Read the model definition and answer for the solid it produces. Units are mm, in the model's axes. A direction names the side the tool comes from. Coordinates: 2 decimals unless noted, no trailing zeros. Write each loop counter-clockwise with the first axis right and the second up, starting at its lowest first coordinate (ties: lowest second). Pieces come first, ordered by that corner, then holes. Notation, with made-up numbers: (-12.5, 28.25) - (1.5, 28.25) arc R9 cw to (1.5, 45.25) - close; hole circle Ø9 at (43.5, 10.5). An arc over 180 degrees is marked (long way). Return JSON: item names as keys, results as strings.
```python
from build123d import *

# Parameters (mm, degrees)
BOSS_EXTRUDE1_DEPTH        = 2
M3_CLEARANCE_HOLE1_D       = 3.242
HOLE1_D                    = 10.1
SKETCHED_START             = 62.517190459
SKETCHED_BEND1_OUTLINE_W   = 2
SKETCHED_BEND1_OUTLINE_H   = 20.000000002
SKETCHED_BEND1_DEPTH       = 31.482809541
SKETCHED_START_2           = 60.939670459
SKETCHED_BEND1_2_OUTLINE_R = 5.05
SKETCHED_BEND1_2_DEPTH     = 0.021621314
SKETCHED_START_3           = 58.939670459
SKETCHED_BEND1_3_OUTLINE_R = 5.05
SKETCHED_BEND1_3_DEPTH     = 4
SKETCHED_START_4           = -10.000000001
SKETCHED_BEND1_4_DEPTH     = 20.000000002
CUT_EXTRUDE1_REACH         = 45.464


with BuildPart() as part:
    # Sketch5 → Boss-Extrude1 (new body)
    with BuildSketch(Plane(origin=(1.681750162, 0, 0), x_dir=(0, -1, 0), z_dir=(-1, 0, 0))):
        with BuildLine():
            Line((-35.93967046, 10.000000001), (-86.258661155, 10.000000001))
            Line((-86.258661155, 10.000000001), (-90.955360298, 5.303300858))
            ThreePointArc((-90.955360298, 5.303300858), (-93.152059438, 0), (-90.955360298, -5.303300858))
            Line((-90.955360298, -5.303300858), (-86.258661155, -10.000000001))
            Line((-86.258661155, -10.000000001), (-35.93967046, -10.000000001))
            ThreePointArc((-35.93967046, -10.000000001), (-33.818350116, -9.121320344), (-32.93967046, -7.000000001))
            Line((-32.93967046, -7.000000001), (-32.93967046, 7.000000001))
            ThreePointArc((-32.93967046, 7.000000001), (-33.818350116, 9.121320344), (-35.93967046, 10.000000001))
        make_face()
    extrude(amount=-BOSS_EXTRUDE1_DEPTH)

    # M3 Clearance Hole1 (through all)
    with Locations(Plane(origin=(3.681750162, 0, 0), x_dir=(0, 0, -1), z_dir=(1, 0, 0))):
        with Locations((0, 40.439670459), (0, 55.439670459)):
            Hole(M3_CLEARANCE_HOLE1_D / 2)

    # Hole1 (through all)
    with Locations(Plane.ZY.offset(-1.681750162)):
        with Locations((0, 85.65205944)):
            Hole(HOLE1_D / 2)

    # Sketched Bend1: read off the stored shape, not the designer's step
    # Sketched Bend1 outline → Sketched Bend1 (cut)
    with BuildSketch(Plane(origin=(0, 0, 0), x_dir=(1, 0, 0), z_dir=(0, 1, 0)).offset(SKETCHED_START)):
        with Locations((2.681750162, 0)):
            Rectangle(SKETCHED_BEND1_OUTLINE_W, SKETCHED_BEND1_OUTLINE_H)
    extrude(amount=SKETCHED_BEND1_DEPTH, mode=Mode.SUBTRACT)

    # Sketched Bend1 2 outline → Sketched Bend1 2 (add)
    with BuildSketch(Plane(origin=(0, 0, 0), x_dir=(1, 0, 0), z_dir=(0, 1, 0)).offset(SKETCHED_START_2)):
        with BuildLine():
            Line((1.681750162, 10.000000001), (-22.924851553, 10.000000001))
            Line((-22.924851553, 10.000000001), (-27.621550696, 5.303300858))
            ThreePointArc((-27.621550696, 5.303300858), (-29.818249837, 0), (-27.621550696, -5.303300858))
            Line((-27.621550696, -5.303300858), (-22.924851553, -10.000000001))
            Line((-22.924851553, -10.000000001), (1.681750162, -10.000000001))
            Line((1.681750162, -10.000000001), (1.681750162, 10.000000001))
        make_face()
        with Locations((-22.318249838, 0)):
            Circle(SKETCHED_BEND1_2_OUTLINE_R, mode=Mode.SUBTRACT)
    extrude(amount=SKETCHED_BEND1_2_DEPTH)

    # Sketched Bend1 3 outline → Sketched Bend1 3 (add)
    with BuildSketch(Plane(origin=(0, 0, 0), x_dir=(1, 0, 0), z_dir=(0, 1, 0)).offset(SKETCHED_START_3)):
        with BuildLine():
            Line((1.681750162, 10.000000001), (-22.924851553, 10.000000001))
            Line((-22.924851553, 10.000000001), (-27.621550696, 5.303300858))
            ThreePointArc((-27.621550696, 5.303300858), (-29.818249837, 0), (-27.621550696, -5.303300858))
            Line((-27.621550696, -5.303300858), (-22.924851553, -10.000000001))
            Line((-22.924851553, -10.000000001), (1.681750162, -10.000000001))
            Line((1.681750162, -10.000000001), (1.681750162, 10.000000001))
        make_face()
        with Locations((-22.318249838, 0)):
            Circle(SKETCHED_BEND1_3_OUTLINE_R, mode=Mode.SUBTRACT)
    extrude(amount=SKETCHED_BEND1_3_DEPTH)

    # Sketched Bend1 4 outline → Sketched Bend1 4 (cut)
    with BuildSketch(Plane.XY.offset(SKETCHED_START_4)):
        with BuildLine():
            Line((-0.318249838, 60.939670459), (-31, 60.939670459))
            Line((-31, 60.939670459), (-31, 58.939670459))
            Line((-31, 58.939670459), (1.681750162, 58.939670459))
            ThreePointArc((1.681750162, 58.939670459), (1.095963724, 60.353884021), (-0.318249838, 60.939670459))
        make_face()
        with BuildLine():
            Line((-31, 64), (-31, 62.939670452))
            Line((-31, 62.939670452), (-0.318249838, 62.939670459))
            ThreePointArc((-0.318249838, 62.939670459), (2.510177287, 61.768097584), (3.681750162, 58.939670459))
            Line((3.681750162, 58.939670459), (3.681750162, 62.517190459))
            Line((3.681750162, 62.517190459), (1.681750162, 62.517190459))
            Line((1.681750162, 62.517190459), (1.681750162, 64))
            Line((1.681750162, 64), (-31, 64))
        make_face()
    extrude(amount=SKETCHED_BEND1_4_DEPTH, mode=Mode.SUBTRACT)

    # Sketch15 → Cut-Extrude1 (cut, up to next)
    with BuildSketch(Plane(origin=(0, 62.939670459, 0), x_dir=(1, 0, 0), z_dir=(0, 1, 0)), mode=Mode.PRIVATE) as cut_extrude1_sk1:
        with BuildLine():
            Line((-21.068249838, 9.000000001), (-21.068249838, 10.000000001))
            Line((-21.068249838, 10.000000001), (-22.924851553, 10.000000001))
            Line((-22.924851553, 10.000000001), (-23.568249838, 9.356601716))
            Line((-23.568249838, 9.356601716), (-23.568249838, 9.000000001))
            Line((-23.568249838, 9.000000001), (-22.943249838, 8.375000001))
            ThreePointArc((-22.943249838, 8.375000001), (-22.318249838, 8.116116524), (-21.693249838, 8.375000001))
            Line((-21.693249838, 8.375000001), (-21.068249838, 9.000000001))
        make_face()
    cut_extrude1_tool1 = extrude(cut_extrude1_sk1.sketch, amount=-CUT_EXTRUDE1_REACH, mode=Mode.PRIVATE) & part.part
    # Sketch15 → Cut-Extrude1 (cut, up to next)
    with BuildSketch(Plane(origin=(0, 62.939670459, 0), x_dir=(1, 0, 0), z_dir=(0, 1, 0)), mode=Mode.PRIVATE) as cut_extrude1_sk2:
        with BuildLine():
            Line((-21.068249838, -9.000000001), (-21.693249838, -8.375000001))
            ThreePointArc((-21.693249838, -8.375000001), (-22.318249838, -8.116116524), (-22.943249838, -8.375000001))
            Line((-22.943249838, -8.375000001), (-23.568249838, -9.000000001))
            Line((-23.568249838, -9.000000001), (-23.568249838, -9.356601716))
            Line((-23.568249838, -9.356601716), (-22.924851553, -10.000000001))
            Line((-22.924851553, -10.000000001), (-21.068249838, -10.000000001))
            Line((-21.068249838, -10.000000001), (-21.068249838, -9.000000001))
        make_face()
    cut_extrude1_tool2 = extrude(cut_extrude1_sk2.sketch, amount=-CUT_EXTRUDE1_REACH, mode=Mode.PRIVATE) & part.part
    add(cut_extrude1_tool1.solids().sort_by_distance((-22.260131, 62.93967, -9.16246))[0], mode=Mode.SUBTRACT)
    add(cut_extrude1_tool2.solids().sort_by_distance((-22.260131, 62.93967, 9.16246))[0], mode=Mode.SUBTRACT)


solid = part.part
```
(1) Flat-ended cylindrical pins translate along their axes: P1, Ø1.1, axis at y = 62, z = 9.5, coming from the -X side; P2, Ø6, axis at y = 44, z = -1.5, coming from the -X side; P3, Ø2, axis at x = -5.5, z = 6.5, coming from the -Y side. Find the tip coordinate at first contact, or state that the pin passes through.
Answer:
{"P1": "x = -23.97", "P2": "x = 1.68", "P3": "y = 60.94"}
(2) A cutting plane is placed at C-C (z = 3.5). Determine the outline of the cut face in (x, y).
Answer:
{"outline": "(-28.95, 60.94) - (-25.96, 60.94) - (-25.96, 62.94) - (-28.95, 62.94) - close; (-18.68, 60.94) - (-0.32, 60.94) arc R2 cw to (1.68, 58.94) - (1.68, 32.94) - (3.68, 32.94) - (3.68, 58.94) arc R4 ccw to (-0.32, 62.94) - (-18.68, 62.94) - close"}
(3) A cutting plane is placed at D-D (y = 43). Determine the outline of the cut face in (x, z).
Answer:
{"outline": "(1.68, -10) - (3.68, -10) - (3.68, 10) - (1.68, 10) - close"}
(4) Which of the six approach directions +Z, -Z, +X, -X, +Y, -Y give full straight-line access (tool end or side, diameter ignored) to faces 5 (the face through (-25.623, 61.926, 7.302)), 6 (the face through (-21.068, 62, 9.5))?
Answer:
{"face 5": "+Z, -X, +Y, -Y", "face 6": "+Z, +Y, -Y"}
(5) Straight lines are drawn through the part: line 1 (Y direction, x = 2.15, z = 0); line 2 (Y direction, x = -17, z = 3); line 3 (X direction, y = 53.5, z = 5.5). For each, find the intervals that lie inside material, in ascending order. Write a range as from..to.
Answer:
{"line 1": "32.94..38.82, 42.06..53.82, 57.06..62.09", "line 2": "60.94..62.94", "line 3": "1.68..3.68"}
(6) A cutting plane is placed at B-B (x = -26). Determine the outline of the cut face in (y, z).
Answer:
{"outline": "(60.94, -6.92) - (62.94, -6.92) - (62.94, -3.46) - (60.94, -3.46) - close; (60.94, 3.46) - (62.94, 3.46) - (62.94, 6.92) - (60.94, 6.92) - close"}
(7) Determine the mould class of faces 1 (the face through (2.668, 38.857, -0.351)), 2 (the face through (-22.328, 61.954, -8.116)), 3 (the face through (-21.068, 62, -9.5)), 4 (the face through (1.682, 46, 0)) for opening direction X: +X half, -X half, draft (parallel to the pull), parting line (faces both ways), or undercut.
Answer:
{"face 1": "draft", "face 2": "undercut", "face 3": "undercut", "face 4": "-X half"}
(8) A cutting plane is placed at A-A (z = 0). Determine the outline of the cut face in (x, y), and give its area (3 significant figures).
Answer:
{"outline": "(-29.82, 60.94) - (-27.37, 60.94) - (-27.37, 62.94) - (-29.82, 62.94) - close; (-17.27, 60.94) - (-0.32, 60.94) arc R2 cw to (1.68, 58.94) - (1.68, 57.06) - (3.68, 57.06) - (3.68, 58.94) arc R4 ccw to (-0.32, 62.94) - (-17.27, 62.94) - close; (1.68, 32.94) - (3.68, 32.94) - (3.68, 38.82) - (1.68, 38.82) - close; (1.68, 42.06) - (3.68, 42.06) - (3.68, 53.82) - (1.68, 53.82) - close", "area": "87.3 mm²"}
